Can you work these out from the model? Positions are in its coordinate system, mm. Face numbers are marked on the shaded views. A direction names the side the tool comes from. Give positions to 0.01 mm unless a question says otherwise; leave off trailing zeros. Loops run counter-clockwise (first coordinate to the right, second up) from the corner with the lowest first, then second, coordinate; pieces in that order, holes last. Notation, with made-up numbers: M 21,20.25 L 47,20.25 A22 cw 47,38.25 Z; hole C 31.25,47 d1. An arc over 180 degrees is marked long. One line per item, written item: value. Start each with the question number.
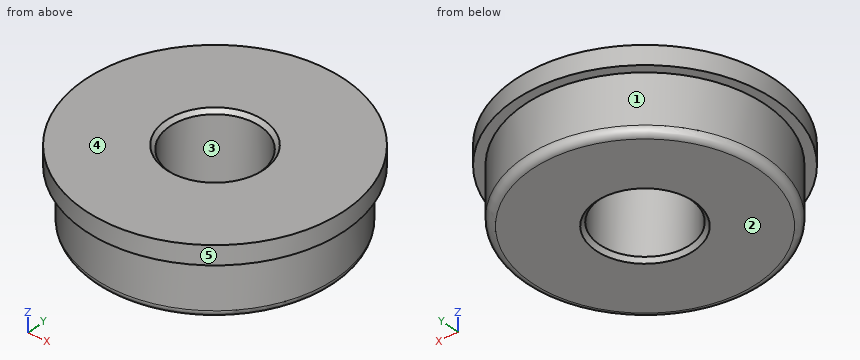
from build123d import *

# Parameters (mm, degrees)
SKETCH_1_R      = 16
SKETCH_1_R_2    = 6
EXTRUDE_1_DEPTH = 5
SKETCH_2_R      = 17.25
SKETCH_2_R_2    = 16
EXTRUDE_2_DEPTH = 2.5
CHAMFER_1_SIZE  = 0.5
FILLET_1_R      = 1


with BuildPart() as part:
    # 草图1 → 凸台-拉伸1 (new, symmetric)
    with BuildSketch(Plane.XY):
        Circle(SKETCH_1_R)
        Circle(SKETCH_1_R_2, mode=Mode.SUBTRACT)
    extrude(amount=EXTRUDE_1_DEPTH, both=True)

    # 草图2 → 凸台-拉伸2 (add)
    with BuildSketch(Plane.XY.offset(5)):
        Circle(SKETCH_2_R)
        Circle(SKETCH_2_R_2, mode=Mode.SUBTRACT)
    extrude(amount=-EXTRUDE_2_DEPTH)

    # 倒角1
    chamfer_1_edges = [part.edges().sort_by_distance(p)[0] for p in [
        (-6, 0, -5),
        (-6, 0, 5),
    ]]
    chamfer(chamfer_1_edges, length=CHAMFER_1_SIZE)

    # 圆角1
    fillet_1_edges = [part.edges().sort_by_distance(p)[0] for p in [
        (-16, 0, -5),
    ]]
    fillet(fillet_1_edges, radius=FILLET_1_R)


solid = part.part
Q1. Which directions (+Z, -Z, +X, -X, +Y, -Y) give clear straight access to the entire face, cutting with the end or side of a thin tool? Please do the marked faces 1 and 2.
Q2. If we mould it in two halves opening along X, with no side actions, what happens to the marked faces 3, 4 and 5? For each: released by +X, released by -X, zero draft, split by the parting line, or undercut.
Q3. If we section it at C-C, the plane z = -1: Write out the boundary of the cut face in (x, y), plus the area to 3 significant figures.
Q4. I need wall thicknesses on line 1 along Y through (x, z) = (0, -0.5); line 2 along Y through (x, z) = (0, 4.25); line 3 along X through (y, z) = (2.5, 1.5). Which ranges of each line are inside material? Lowest first, please.
Q5. For P1, Ø3, axis at x = 6, z = 0.5, coming from the -Y side; P2, Ø4, axis at y = -10.5, z = 1.5, coming from the -X side; P3, Ø6, axis at x = 1, z = -1.5, coming from the -Y side, each with a flat end and sliding along its axis, tell me the tip position at first contact or that it passes through.
Q6. If we section it at A-A, the plane x = 0: Write out the boundary of the cut face in (y, z), plus the area to 3 significant figures.
Response:
1. face 1: -Z
1. face 2: -Z, +X, -X, +Y, -Y
2. face 3: undercut
2. face 4: zero draft
2. face 5: split by the parting line
3. outline: C 0,0 d32; hole C 0,0 d12
3. area: 691 mm^2
4. line 1: -16 to -6, 6 to 16
4. line 2: -17.25 to -6, 6 to 17.25
4. line 3: -15.8 to -5.45, 5.45 to 15.8
5. P1: y = -15.35
5. P2: x = -14.86
5. P3: y = -16
6. outline: M -17.25,2.5 L -16,2.5 L -16,-4 A1 ccw -15,-5 L -6.5,-5 L -6,-4.5 L -6,4.5 L -6.5,5 L -17.25,5 Z; M 6,-4.5 L 6.5,-5 L 15,-5 A1 ccw 16,-4 L 16,2.5 L 17.25,2.5 L 17.25,5 L 6.5,5 L 6,4.5 Z
6. area: 205 mm^2
